Source: three-view drawing plus pictorial views. Frame: mm from the lowest corner of the part. A direction names the side the tool comes from. Give positions to 0.01 mm unless a question says otherwise; leave off trailing zeros. Order: outer loops, then holes, each group sorted by start corner. A loop starts at its lowest first (then second) coordinate and runs counter-clockwise, first axis right, second up.
1) Draft query along X for the marked faces 3, 4, 5 and 6. Return one class per face: released by +X, released by -X, zero draft, split by the parting line, or undercut.
2) Section D-D, the plane y = 65. Return loops of the section in (x, z).
3) Section B-B, the plane y = 13.5. Return loops of the section in (x, z), plus the area to 3 significant figures.
4) Section A-A, the plane z = 5. Return loops of the section in (x, y), plus the area to 3 significant figures.
5) Access query for the marked faces 1 and 2. Directions: +Z, -Z, +X, -X, +Y, -Y. A direction counts if a zero-diameter tool reaches every point of the face in a straight line with its end or side. Return the directions, or none.
6) Section C-C, the plane x = 17. Return loops of the section in (y, z).
7) First-contact query: P1, Ø1, axis at x = 18.5, z = 39, coming from the -Y side; P2, Ø5, axis at x = 18, z = 22.5, coming from the -Y side; P3, Ø17, axis at x = 14, y = 39, coming from the +Z side; P4, Ø11, axis at x = 15, z = 3, coming from the -Y side. Flat tips, straight axial feed; report the tip coordinate or a pass-through.
8) Material intervals for line 1 (X direction, y = 19, z = 4); line 2 (Z direction, x = 24, y = 52); line 3 (Z direction, x = 8.5, y = 35), sorted ascending.
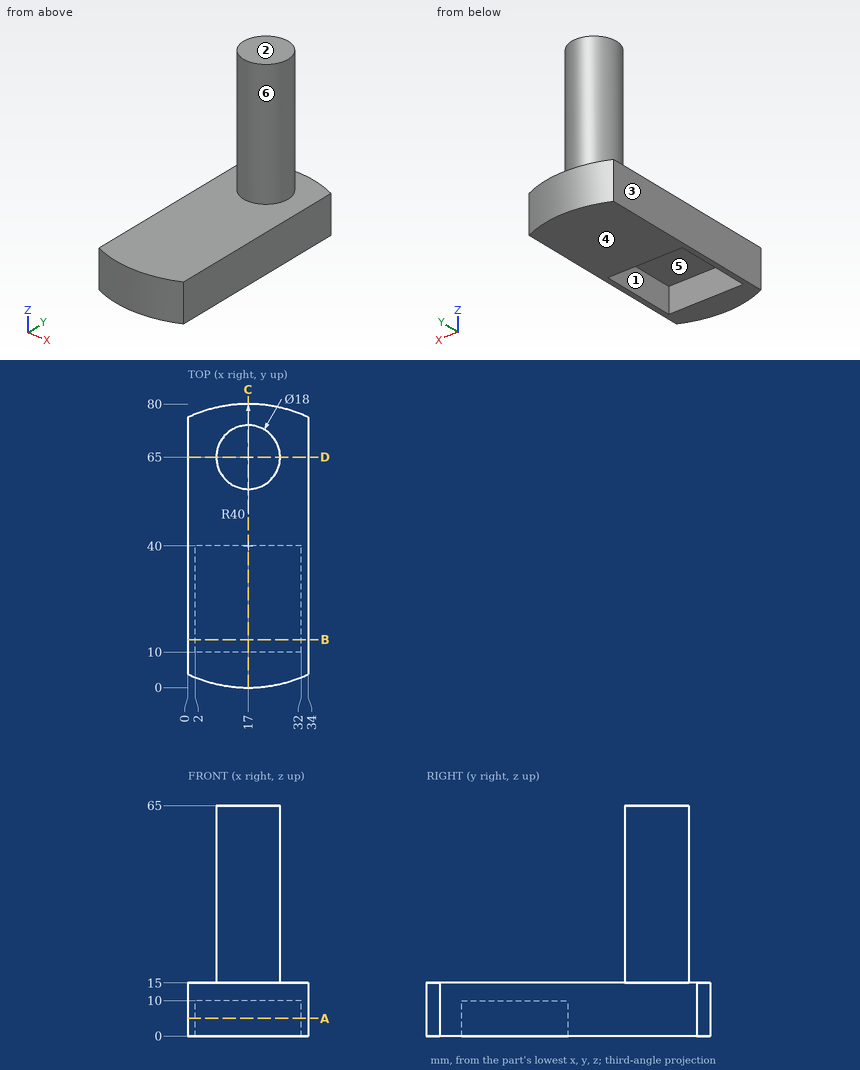
From the geometry:
1. face 3: released by -X
1. face 4: zero draft
1. face 5: undercut
1. face 6: split by the parting line
2. outline: (0, 0) - (34, 0) - (34, 15) - (26, 15) - (26, 65) - (8, 65) - (8, 15) - (0, 15) - close
3. outline: (0, 0) - (2, 0) - (2, 10) - (32, 10) - (32, 0) - (34, 0) - (34, 15) - (0, 15) - close
3. area: 210 mm2
4. outline: (0, 3.79) arc R40 ccw to (34, 3.79) - (34, 76.21) arc R40 ccw to (0, 76.21) - close; hole (2, 10) - (32, 10) - (32, 40) - (2, 40) - close
4. area: 1,740 mm2
5. face 1: -Z
5. face 2: +Z, +X, -X, +Y, -Y
6. outline: (0, 0) - (10, 0) - (10, 10) - (40, 10) - (40, 0) - (80, 0) - (80, 15) - (74, 15) - (74, 65) - (56, 65) - (56, 15) - (0, 15) - close
7. P1: stops at y = 56.06
7. P2: stops at y = 56
7. P3: stops at z = 15
7. P4: stops at y = 0
8. line 1: x = 0 to 2, 32 to 34
8. line 2: z = 0 to 15
8. line 3: z = 10 to 15
